from build123d import *

# Parameters (mm, degrees)
F0_R          = 12.5
F1_DEPTH      = 300
F3_R          = 12.5
F5_R          = 12.5
F6_DEPTH      = 300
F6_DEPTH_BACK = 300


with BuildPart() as f1:
    # F0 (on Front) → F1 (new body, symmetric)
    with BuildSketch(Plane.XZ):
        Circle(F0_R)
    extrude(amount=F1_DEPTH, both=True)

    # F3 (on offset) → F4 (join, up to the next surface of F1)
    with BuildSketch(Plane.YZ.offset(1300)):
        with Locations((-250, 0)):
            Circle(F3_R)
        with Locations((250, 0)):
            Circle(F3_R)
    extrude(until=Until.NEXT, dir=(-1, 0, 0))

    # F5 (on Front) → F6 (join, two sides)
    with BuildSketch(Plane.XZ) as f6_sk:
        with Locations((1300, 0)):
            Circle(F5_R)
    extrude(amount=F6_DEPTH)
    extrude(f6_sk.sketch, amount=-F6_DEPTH_BACK)


solid = f1.part
Read the model definition and answer for the solid it produces. Units are mm, in the model's axes. A direction names the side the tool comes from. Give positions to 0.01 mm unless a question says otherwise; leave off trailing zeros. Write each loop counter-clockwise with the first axis right and the second up, starting at its lowest first coordinate (ties: lowest second). Pieces come first, ordered by that corner, then holes. Notation, with made-up numbers: (25, -34.75) - (81, -34.75) arc R21 ccw to (81, -0.75) - close; hole circle Ø5 at (39, 26). An arc over 180 degrees is marked (long way). Answer in a Markdown table with one row per item. Add a question column.
Item 1: Flat-ended cylindrical pins translate along their axes: P1, Ø5, axis at x = 807, z = -5.5, coming from the -Y side; P2, Ø2, axis at y = -22.5, z = 6, coming from the -X side; P3, Ø3, axis at x = 1149.5, z = 1, coming from the +Y side. Find the tip coordinate at first contact, or state that the pin passes through.
Item 2: Section A-A, the plane z = 0 is taken. Write down the section's boundary in (x, y).
Item 3: Section B-B, the plane y = 197.5 is taken. Write down the section's boundary in (x, z).
Item 4: Section C-C, the plane x = 451.5 is taken. Write down the section's boundary in (y, z).
Item 5: Find the intervals of material crossed by L1, parallel to Y at x = 831, z = 2.5; L2, parallel to Y at x = 472, z = -1.25; L3, parallel to Z at x = 121.5, y = -248.5, in increasing order.
Item 6: Determine the mould class of faces 3 (the face through (659.1, -238.077, 3.755)), 4 (the face through (0, 300, 0)), 5 (the face through (1300, -300, 0)) for opening direction Y: pulls with the +Y half, pulls with the -Y half, needs draft (parallel to the pull), parting line crosses it, or undercut.
Item 7: A tool of negligible diameter and unlimited length cuts with its end or side. For faces 1 (the face through (659.1, 261.923, 3.755)), 2 (the face through (0, -300, 0)), from which of +Z, -Z, +X, -X, +Y, -Y can it reach the whole face along a straight path? Write none if from no direction.
Recorded:
| question | item | result |
|---|---|---|
| 1 | P1 | stops at y = -262.13 |
| 1 | P2 | stops at x = -11.46 |
| 1 | P3 | stops at y = 262.5 |
| 2 | outline | (-12.5, -300) - (12.5, -300) - (12.5, -262.5) - (1287.5, -262.5) - (1287.5, -300) - (1312.5, -300) - (1312.5, 300) - (1287.5, 300) - (1287.5, 262.5) - (12.5, 262.5) - (12.5, 300) - (-12.5, 300) - close; hole (12.5, -237.5) - (1287.5, -237.5) - (1287.5, 237.5) - (12.5, 237.5) - close |
| 3 | outline | circle Ø25 at (0, 0); circle Ø25 at (1300, 0) |
| 4 | outline | circle Ø25 at (-250, 0); circle Ø25 at (250, 0) |
| 5 | L1 | y = -262.25 to -237.75, 237.75 to 262.25 |
| 5 | L2 | y = -262.44 to -237.56, 237.56 to 262.44 |
| 5 | L3 | z = -12.41 to 12.41 |
| 6 | face 3 | undercut |
| 6 | face 4 | pulls with the +Y half |
| 6 | face 5 | pulls with the -Y half |
| 7 | face 1 | none |
| 7 | face 2 | +Z, -Z, +X, -X, -Y |
